Source: CAD feature listing. Evaluate the final solid. Frame: model axes, mm. Round coordinates to 2 decimals unless told otherwise and drop trailing zeros. Loops run counter-clockwise (first coordinate to the right, second up) from the corner with the lowest first, then second, coordinate; pieces in that order, holes last. Notation, with made-up numbers: (70, 44) - (125, 44) arc R26 ccw to (125, 67) - close; hole circle Ø6 at (-21, 87). An arc over 180 degrees is marked (long way). One line per question, with ' | ' between items. Start each with the question number.
1. Cut plane D-D (y = -11). Return loops of the section in (x, z).
2. Ray query, line 1 (X direction, y = 34, z = 1.65); line 2 (X direction, y = 31, z = 2.9); line 3 (X direction, y = -39, z = 3.35). Return the intervals inside material, ascending.
3. Cut plane C-C (z = 2.6). State how many separate pieces and enclosed holes the cut face has, then the cut area to 3 significant figures.
4. Cut plane A-A (x = 31.5). Return loops of the section in (y, z).
5. Pin query (flat end, axial travel): pin 1 (0.8 mm diameter, centred on x = -46.5, z = 2, fed in from +Y); pin 2 (1.2 mm diameter, centred on x = -46, z = 3, fed in from -Y); pin 3 (1.2 mm diameter, centred on y = -43, z = 2, fed in from +X). Return the tip coordinate at first contact, or that it passes through.
6. Cut plane B-B (y = 39). Return loops of the section in (x, z), then the cut area to 3 significant figures.
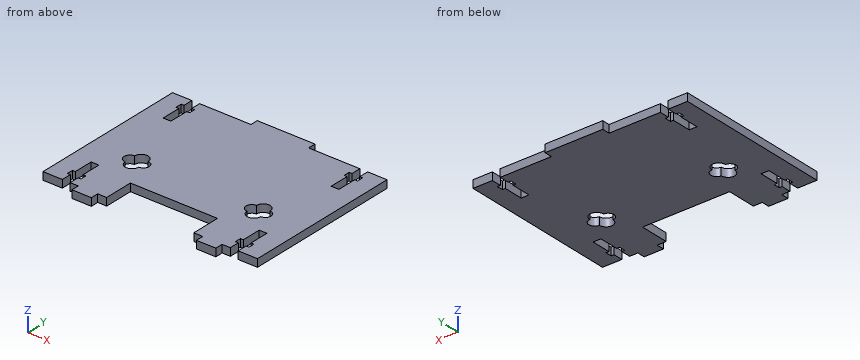
```python
from build123d import *

# Parameters (mm, degrees)
SKETCH1_W           = 110.8
SKETCH1_H           = 82
BOSS_EXTRUDE1_DEPTH = 4
CUT_EXTRUDE1_DEPTH  = 10
SKETCH3_W           = 45
SKETCH3_H           = 15
CUT_EXTRUDE2_DEPTH  = 10
CUT_EXTRUDE3_DEPTH  = 10
SKETCH8_W           = 29.8
SKETCH8_H           = 4
BOSS_EXTRUDE2_DEPTH = 4
SKETCH9_W           = 10
SKETCH9_H           = 4
BOSS_EXTRUDE3_DEPTH = 4


with BuildPart() as part:
    # Sketch1 → Boss-Extrude1 (new body)
    with BuildSketch(Plane.XY):
        Rectangle(SKETCH1_W, SKETCH1_H)
    extrude(amount=BOSS_EXTRUDE1_DEPTH)

    # Sketch2 → Cut-Extrude1 (cut)
    with BuildSketch(Plane.XY.offset(4)):
        Polygon((41.4, -32.8), (41.4, -22.8), (45.4, -22.8), (45.4, -32.8), (46.9, -32.8), (46.9, -36), (45.4, -36), (45.4, -41), (41.4, -41), (41.4, -36), (39.9, -36), (39.9, -32.8), align=None)
        Polygon((-41.4, 32.8), (-41.4, 22.8), (-45.4, 22.8), (-45.4, 32.8), (-46.9, 32.8), (-46.9, 36), (-45.4, 36), (-45.4, 41), (-41.4, 41), (-41.4, 36), (-39.9, 36), (-39.9, 32.8), align=None)
        Polygon((45.4, 22.8), (45.4, 32.8), (46.9, 32.8), (46.9, 36), (45.4, 36), (45.4, 41), (41.4, 41), (41.4, 36), (39.9, 36), (39.9, 32.8), (41.4, 32.8), (41.4, 22.8), align=None)
        Polygon((-45.4, -22.8), (-45.4, -32.8), (-46.9, -32.8), (-46.9, -36), (-45.4, -36), (-45.4, -41), (-41.4, -41), (-41.4, -36), (-39.9, -36), (-39.9, -32.8), (-41.4, -32.8), (-41.4, -22.8), align=None)
    extrude(amount=-CUT_EXTRUDE1_DEPTH, mode=Mode.SUBTRACT)

    # Sketch3 → Cut-Extrude2 (cut)
    with BuildSketch(Plane.XY.offset(4)):
        with Locations((0, -33.5)):
            Rectangle(SKETCH3_W, SKETCH3_H)
    extrude(amount=-CUT_EXTRUDE2_DEPTH, mode=Mode.SUBTRACT)

    # Sketch6 → Cut-Extrude3 (cut)
    with BuildSketch(Plane.XY.offset(4)):
        with BuildLine():
            ThreePointArc((-35.03018163, -13.984149147), (-31.5, -17.463580565), (-27.96981837, -13.984149147))
            ThreePointArc((-27.96981837, -13.984149147), (-25.015698228, -11), (-27.96981837, -8.015850853))
            ThreePointArc((-27.96981837, -8.015850853), (-31.5, -4.536419435), (-35.03018163, -8.015850853))
            ThreePointArc((-35.03018163, -8.015850853), (-37.984301772, -11), (-35.03018163, -13.984149147))
        make_face()
        with BuildLine():
            ThreePointArc((27.96981837, -13.984149147), (25.015698228, -11), (27.96981837, -8.015850853))
            ThreePointArc((27.96981837, -8.015850853), (31.5, -4.536419435), (35.03018163, -8.015850853))
            ThreePointArc((35.03018163, -8.015850853), (37.984301772, -11), (35.03018163, -13.984149147))
            ThreePointArc((35.03018163, -13.984149147), (31.5, -17.463580565), (27.96981837, -13.984149147))
        make_face()
    extrude(amount=-CUT_EXTRUDE3_DEPTH, mode=Mode.SUBTRACT)

    # Sketch8 → Boss-Extrude2 (add)
    with BuildSketch(Plane.XY.offset(4)):
        with Locations((0, 43)):
            Rectangle(SKETCH8_W, SKETCH8_H)
    extrude(amount=-BOSS_EXTRUDE2_DEPTH)

    # Sketch9 → Boss-Extrude3 (add)
    with BuildSketch(Plane.XY.offset(4)):
        with Locations((-32.15, -43)):
            Rectangle(SKETCH9_W, SKETCH9_H)
        with Locations((32.15, -43)):
            Rectangle(SKETCH9_W, SKETCH9_H)
    extrude(amount=-BOSS_EXTRUDE3_DEPTH)


solid = part.part
```
Answers follow:
1) outline: (-55.4, 0) - (-37.98, 0) - (-37.98, 4) - (-55.4, 4) - close; (-25.02, 0) - (25.02, 0) - (25.02, 4) - (-25.02, 4) - close; (37.98, 0) - (55.4, 0) - (55.4, 4) - (37.98, 4) - close
2) line 1: x = -55.4 to -46.9, -39.9 to 39.9, 46.9 to 55.4 | line 2: x = -55.4 to -45.4, -41.4 to 41.4, 45.4 to 55.4 | line 3: x = -55.4 to -45.4, -41.4 to -22.5, 22.5 to 41.4, 45.4 to 55.4
3) separate pieces: 1 | enclosed holes: 2 | area: 8,060 mm2
4) outline: (-45, 0) - (-17.46, 0) - (-17.46, 4) - (-45, 4) - close; (-4.54, 0) - (41, 0) - (41, 4) - (-4.54, 4) - close
5) pin 1: stops at y = 41 | pin 2: stops at y = -41 | pin 3: stops at x = 37.15
6) outline: (-55.4, 0) - (-45.4, 0) - (-45.4, 4) - (-55.4, 4) - close; (-41.4, 0) - (41.4, 0) - (41.4, 4) - (-41.4, 4) - close; (45.4, 0) - (55.4, 0) - (55.4, 4) - (45.4, 4) - close | area: 411 mm2
